The listing builds one solid part. Answer for the finished solid, in the listing's coordinates (mm). A direction names the side the tool comes from. Give positions to 0.01 mm unless a question says otherwise; leave off trailing zeros. Order: outer loops, then holes, each group sorted by start corner. A loop starts at its lowest first (then second) coordinate and runs counter-clockwise, first axis right, second up. Notation, with made-up numbers: (-35, 57) - (19, 57) arc R22 ccw to (19, 65) - close; hole circle Ø2 at (15.5, -2.75). An arc over 180 degrees is marked (long way). Answer as a JSON object with one key per item and string values. Group by question number.
Q1. Given pin 1 (8 mm diameter, centred on y = -11, z = -10.5, fed in from +X); pin 2 (4.5 mm diameter, centred on x = -94.3, z = -22.5, fed in from +Y); pin 3 (1.5 mm diameter, centred on y = -12.5, z = -36.5, fed in from +X); pin 4 (8 mm diameter, centred on x = -106, y = 4.5, fed in from -Z), each flat-ended and moving along its own axis, determine where each tip first touches the part or whether it passes through.
Q2. A cutting plane is placed at A-A, the plane z = -6.5. Give the vertices of the cut face in (x, y).
Q3. A cutting plane is placed at B-B, the plane z = -18. Give the vertices of the cut face in (x, y).
Q4. The mould has two halves that part along Z. Classify faces 1 (the face through (-92.6, -20.9, -20.6)), 2 (the face through (0, -11, -31)), 3 (the face through (-112, -11, -39)): released by +Z, released by -Z, zero draft, split by the parting line, or undercut.
Q5. Consider line 1 (X direction, y = -21.8, z = -22.5); line 2 (Z direction, x = -38, y = -20); line 3 (X direction, y = -20, z = -22). Determine where each line is inside the solid, lowest interval first.
Q6. For faces 4 (the face through (-126.8, -12.1, -36.5)), 5 (the face through (-36.748, -20.884, -24.524)), 6 (the face through (-131.301, -3, 7)), 7 (the face through (-131.301, -2, -36)), determine the directions among +Z, -Z, +X, -X, +Y, -Y from which every point of the face is accessible in a straight line to the end or side of a thin tool.
from build123d import *

# Parameters (mm, degrees)
BOSS_EXTRUDE1_DEPTH  = 5
BOSS_EXTRUDE3_DEPTH  = 29
SKETCH7_R            = 2.55
CUT_EXTRUDE1_DEPTH   = 4
BOSS_EXTRUDE4_DEPTH  = 5
CUT_EXTRUDE2_DEPTH   = 50
BOSS_EXTRUDE5_DEPTH  = 39
BOSS_EXTRUDE6_DEPTH  = 5
BOSS_EXTRUDE7_DEPTH  = 5
BOSS_EXTRUDE8_DEPTH  = 5
FILLET1_START        = -96.499038859
FILLET1_DEPTH        = 93.561345122
FILLET1_2_ANGLE      = 90
BOSS_EXTRUDE9_DEPTH  = 5
FILLET2_R            = 10
FILLET3_R            = 5
FILLET4_R            = 2
BOSS_EXTRUDE10_START = 5
BOSS_EXTRUDE10_DEPTH = 5
FILLET5_R            = 10
BOSS_EXTRUDE11_DEPTH = 5
FILLET6_R            = 10
FILLET7_R            = 5
FILLET8_R            = 2


with BuildPart() as part:
    # Sketch1 → Boss-Extrude1 (new body)
    with BuildSketch(Plane.XY):
        Polygon((0, 0), (-101.301402794, 27.143629071), (-101.301402794, -22.856370929), (0, -22.856370929), align=None)
    extrude(amount=BOSS_EXTRUDE1_DEPTH)

    # Sketch3 → Boss-Extrude3 (add)
    with BuildSketch(Plane(origin=(0, 0, 0), x_dir=(-1, 0, 0), z_dir=(0, 0, -1))):
        Polygon((101.301402794, 27.143629071), (101.301402794, -22.856370929), (28.3, -22.856370929), (28.3, 0), (0, 0), align=None)
    extrude(amount=BOSS_EXTRUDE3_DEPTH)

    # Sketch7 → Cut-Extrude1 (cut)
    with BuildSketch(Plane.XZ.offset(22.856370929)):
        with Locations(Location((-38.3, -6.5, 0), (0, 0, 270))):
            Circle(SKETCH7_R)
        with Locations(Location((-38.3, -22.5, 0), (0, 0, 90))):
            Circle(SKETCH7_R)
        with Locations(Location((-94.302805589, -22.5, 0), (0, 0, 270))):
            Circle(SKETCH7_R)
        with Locations(Location((-94.302805589, -6.5, 0), (0, 0, 90))):
            Circle(SKETCH7_R)
    extrude(amount=-CUT_EXTRUDE1_DEPTH, mode=Mode.SUBTRACT)

    # Sketch8 → Boss-Extrude4 (add)
    with BuildSketch(Plane(origin=(0, 0, -29), x_dir=(-1, 0, 0), z_dir=(0, 0, -1))):
        Polygon((0, 0), (0, -22.856370929), (28.3, -22.856370929), (101.301402794, -22.856370929), (101.301402794, 27.143629071), align=None)
    extrude(amount=BOSS_EXTRUDE4_DEPTH)

    # Sketch9 → Cut-Extrude2 (cut)
    with BuildSketch(Plane(origin=(0, 0, -34), x_dir=(-1, 0, 0), z_dir=(0, 0, -1))):
        Polygon((101.301402794, 27.143629071), (29.621530414, 7.937065153), (101.301402794, -5.041318946), align=None)
    extrude(amount=-CUT_EXTRUDE2_DEPTH, mode=Mode.SUBTRACT)

    # Sketch10 → Boss-Extrude5 (add)
    with BuildSketch(Plane.XY.offset(5)):
        Polygon((-101.301402794, -22.856370929), (-136.301402794, -22.856370929), (-136.301402794, 12.143629071), (-101.301402794, -5.041318946), align=None)
    extrude(amount=-BOSS_EXTRUDE5_DEPTH)

    # Sketch11 → Boss-Extrude6 (add)
    with BuildSketch(Plane.XY.offset(5)):
        Polygon((-136.301402794, -22.856370929), (-131.301402794, -22.856370929), (-131.301402794, 18.143473933), (-136.301402794, 24.143629071), align=None)
    extrude(amount=BOSS_EXTRUDE6_DEPTH)

    # Sketch12 → Boss-Extrude7 (add)
    with BuildSketch(Plane(origin=(0, 0, -34), x_dir=(-1, 0, 0), z_dir=(0, 0, -1))):
        Polygon((136.301402794, -22.856370929), (136.301402794, 24.143629071), (131.301402794, 18.143473933), (131.301402794, -22.856370929), align=None)
    extrude(amount=BOSS_EXTRUDE7_DEPTH)

    # Sketch13 → Boss-Extrude8 (add)
    with BuildSketch(Plane.XY.offset(5)):
        with BuildLine():
            ThreePointArc((0, -22.856370929), (-7.32233047, -5.178701399), (-25, 2.143629071))
            Line((-25, 2.143629071), (-94.318764812, -7.598487996))
            Line((-94.318764812, -7.598487996), (-94.318764812, -22.261326085))
            ThreePointArc((-94.318764812, -22.261326085), (-91.360881343, -22.707239046), (-88.373294914, -22.856370929))
            Line((-88.373294914, -22.856370929), (0, -22.856370929))
        make_face()
    extrude(amount=BOSS_EXTRUDE8_DEPTH)

    # Fillet1: read off the stored shape, not the designer's step
    # Fillet1 outline → Fillet1 (cut)
    with BuildSketch(Plane(origin=(0, 0, 0), x_dir=(-0.13917310096006896, 0.9902680687415698, 0), z_dir=(0.9902680687415698, 0.13917310096006896, 0)).offset(FILLET1_START)):
        with BuildLine():
            ThreePointArc((-3.058159094, 10), (1.941840906, 8.660254038), (5.602094944, 5))
            Line((5.602094944, 5), (5.602094944, 10))
            Line((5.602094944, 10), (-3.058159094, 10))
        make_face()
    extrude(amount=FILLET1_DEPTH, mode=Mode.SUBTRACT)

    # Fillet1 2 outline → Fillet1 2 (revolve, cut)
    with BuildSketch(Plane(origin=(-25, -22.856370929, 0), x_dir=(1, 0, 0), z_dir=(0, -1, 0))):
        with BuildLine():
            Line((25, 10), (16.339745962, 10))
            ThreePointArc((16.339745962, 10), (21.339745962, 8.660254038), (25, 5))
            Line((25, 5), (25, 10))
        make_face()
    revolve(axis=Axis((-25, -22.856370929, 0), (0, 0, 1)), revolution_arc=FILLET1_2_ANGLE, mode=Mode.SUBTRACT)

    # Sketch14 → Boss-Extrude9 (add)
    with BuildSketch(Plane.XY.offset(5)):
        Polygon((-128.991070269, 10.697688119), (-95.669410429, -5.689032412), (-95.669410429, -21.784370313), (-128.991070269, -13.724945051), align=None)
    extrude(amount=BOSS_EXTRUDE9_DEPTH)

    # Fillet2
    fillet2_edges = [part.edges().sort_by_distance(p)[0] for p in [
        (-128.991070269, -13.724945051, 7.5),
    ]]
    fillet(fillet2_edges, radius=FILLET2_R)

    # Fillet3
    fillet3_edges = [part.edges().sort_by_distance(p)[0] for p in [
        (-112.330240349, 2.504327853, 10),
    ]]
    fillet(fillet3_edges, radius=FILLET3_R - 0.0001)  # a hair under: the kernel refuses the full size

    # Fillet4
    fillet4_edges = [part.edges().sort_by_distance(p)[0] for p in [
        (-95.669410429, -21.784370313, 7.5),
    ]]
    fillet(fillet4_edges, radius=FILLET4_R)

    # Sketch15 → Boss-Extrude10 (add)
    with BuildSketch(Plane(origin=(0, 0, -34), x_dir=(-1, 0, 0), z_dir=(0, 0, -1)).offset(BOSS_EXTRUDE10_START)):
        with BuildLine():
            Line((88.373294914, -22.856370929), (80, -22.856370929))
            Line((80, -22.856370929), (0, -22.856370929))
            ThreePointArc((0, -22.856370929), (7.32233047, -5.178701399), (25, 2.143629071))
            Line((25, 2.143629071), (94.318764812, -7.598487996))
            Line((94.318764812, -7.598487996), (94.318764812, -22.261326085))
            ThreePointArc((94.318764812, -22.261326085), (91.360881343, -22.707239046), (88.373294914, -22.856370929))
        make_face()
    extrude(amount=-BOSS_EXTRUDE10_DEPTH)

    # Fillet5
    # the kernel refuses this fillet: 10 mm, written as the material it takes off along each edge
    with BuildSketch(Plane(origin=(-3.560067398, 5.156815095, -39), x_dir=(0, 0, 1), z_dir=(-0.9902680687415698, -0.13917310096006932, 0))) as fillet5_piece_1:
        with BuildLine():
            CenterArc((10, -8.660254038), FILLET5_R, 120, 60)
            Line((0, -8.660254038), (0, 0))
            Line((0, 0), (5, 0))
        make_face()
    extrude(amount=113.301270189, mode=Mode.SUBTRACT)
    # the kernel refuses this fillet: 10 mm, written as the material it takes off along each edge
    with BuildSketch(Plane(origin=(-25, -22.856370929, -39), x_dir=(0.6477837249350054, -0.7618242879492156, 0), z_dir=(-0.7618242879492156, -0.6477837249350054, 0))) as fillet5_2_piece_1:
        with BuildLine():
            CenterArc((16.339745962, 10), FILLET5_R, 270, 60)
            Line((25, 5), (25, 0))
            Line((25, 0), (16.339745962, 0))
        make_face()
    revolve(axis=Axis((-25, -22.856370929, -39), (0, 0, 1)), revolution_arc=147.330675393, mode=Mode.SUBTRACT)

    # Sketch16 → Boss-Extrude11 (add)
    with BuildSketch(Plane(origin=(0, 0, -34), x_dir=(-1, 0, 0), z_dir=(0, 0, -1))):
        Polygon((128.991070269, 10.697688119), (95.669410429, -5.689032412), (95.669410429, -21.784370313), (128.991070269, -13.724945051), align=None)
    extrude(amount=BOSS_EXTRUDE11_DEPTH)

    # Fillet6
    fillet6_edges = [part.edges().sort_by_distance(p)[0] for p in [
        (-128.991070269, -13.724945051, -36.5),
    ]]
    fillet(fillet6_edges, radius=FILLET6_R)

    # Fillet7
    fillet7_edges = [part.edges().sort_by_distance(p)[0] for p in [
        (-112.330240349, 2.504327853, -39),
    ]]
    fillet(fillet7_edges, radius=FILLET7_R - 0.0001)  # a hair under: the kernel refuses the full size

    # Fillet8
    fillet8_edges = [part.edges().sort_by_distance(p)[0] for p in [
        (-95.669410429, -21.784370313, -36.5),
    ]]
    fillet(fillet8_edges, radius=FILLET8_R)


solid = part.part
Reply:
{
 "1": {"pin 1": "stops at x = -28.3", "pin 2": "stops at y = -3.37", "pin 3": "stops at x = -3.58", "pin 4": "passes through"},
 "2": {"outline": "(-136.3, -22.86) - (-96.85, -22.86) - (-96.85, -18.86) - (-91.75, -18.86) - (-91.75, -22.86) - (-40.85, -22.86) - (-40.85, -18.86) - (-35.75, -18.86) - (-35.75, -22.86) - (-28.3, -22.86) - (-28.3, 0) - (0, 0) - (-29.62, 7.94) - (-101.3, -5.04) - (-136.3, 12.14) - close"},
 "3": {"outline": "(-136.3, -22.86) - (-28.3, -22.86) - (-28.3, 0) - (0, 0) - (-29.62, 7.94) - (-101.3, -5.04) - (-136.3, 12.14) - close"},
 "4": {"face 1": "undercut", "face 2": "zero draft", "face 3": "released by -Z"},
 "5": {"line 1": "x = -136.3 to -96.85, -91.75 to -40.85, -35.75 to -28.3", "line 2": "z = -39 to -25.03, -19.97 to -9.03, -3.97 to 10", "line 3": "x = -136.3 to -96.8, -91.8 to -40.8, -35.8 to -28.3"},
 "6": {"face 4": "-Z, -Y", "face 5": "-Y", "face 6": "+Z, +Y, -Y", "face 7": "-Z, +Y, -Y"}
}
